```python
from build123d import *

# Parameters (mm, degrees)
BOSS_EXTRUDE1_DEPTH = 3
SKETCH2_W           = 78
SKETCH2_H           = 45
CUT_EXTRUDE1_DEPTH  = 10
FILLET1_R           = 10
CUT_EXTRUDE2_DEPTH  = 10


with BuildPart() as part:
    # Sketch1 → Boss-Extrude1 (new body)
    with BuildSketch(Plane(origin=(0, 0, 0), x_dir=(1, 0, 0), z_dir=(0, 1, 0))):
        Polygon((0, 0), (0, 75.000000004), (300, 65), (300, 0), align=None)
    boss_extrude1 = extrude(amount=BOSS_EXTRUDE1_DEPTH)

    # Mirror1: Boss-Extrude1 across Front Plane
    add(boss_extrude1.mirror(Plane.XY))

    # Sketch2 → Cut-Extrude1 (cut)
    with BuildSketch(Plane(origin=(0, 3, 0), x_dir=(1, 0, 0), z_dir=(0, 1, 0))):
        with Locations((55.5, 0)):
            Rectangle(SKETCH2_W, SKETCH2_H)
        with Locations((150, 0)):
            Rectangle(SKETCH2_W, SKETCH2_H)
        with Locations((244.5, 0)):
            Rectangle(SKETCH2_W, SKETCH2_H)
    extrude(amount=-CUT_EXTRUDE1_DEPTH, mode=Mode.SUBTRACT)

    # Fillet1
    fillet1_edges = [part.edges().sort_by_distance(p)[0] for p in [
        (16.5, 1.5, 22.5),
        (16.5, 1.5, -22.5),
        (94.5, 1.5, -22.5),
        (94.5, 1.5, 22.5),
        (111, 1.5, 22.5),
        (111, 1.5, -22.5),
        (189, 1.5, -22.5),
        (189, 1.5, 22.5),
        (205.5, 1.5, 22.5),
        (205.5, 1.5, -22.5),
        (283.5, 1.5, -22.5),
        (283.5, 1.5, 22.5),
    ]]
    fillet(fillet1_edges, radius=FILLET1_R)

    # Sketch3 → Cut-Extrude2 (cut)
    with BuildSketch(Plane(origin=(0, 3, 0), x_dir=(1, 0, 0), z_dir=(0, 1, 0))):
        with BuildLine():
            Line((12, 56.323336113), (12, 44))
            ThreePointArc((12, 44), (14.343145751, 38.343145751), (20, 36))
            Line((20, 36), (280, 36))
            ThreePointArc((280, 36), (285.656854249, 38.343145751), (288, 44))
            Line((288, 44), (288, 47.656669443))
            ThreePointArc((288, 47.656669443), (285.750310824, 53.218496969), (280.266518642, 55.652228699))
            Line((280.266518642, 55.652228699), (20.266518642, 64.318895369))
            ThreePointArc((20.266518642, 64.318895369), (14.438172474, 62.073646937), (12, 56.323336113))
        make_face()
    cut_extrude2 = extrude(amount=-CUT_EXTRUDE2_DEPTH, mode=Mode.SUBTRACT)

    # Mirror2: Cut-Extrude2 across plane
    add(cut_extrude2.mirror(Plane.XY), mode=Mode.SUBTRACT)


solid = part.part
```
Work out the finished part from the listing and answer in its coordinate system (mm). Coordinates: 2 decimals unless noted, no trailing zeros. Loops run counter-clockwise (first coordinate to the right, second up) from the corner with the lowest first, then second, coordinate; pieces in that order, holes last.
1) Section A-A (x = 209.5) is taken. Give the vertices of the cut face in (y, z).
Results:
outline: (0, -68.02) - (3, -68.02) - (3, -58.01) - (0, -58.01) - close; (0, -36) - (3, -36) - (3, -20.5) - (0, -20.5) - close; (0, 20.5) - (3, 20.5) - (3, 36) - (0, 36) - close; (0, 58.01) - (3, 58.01) - (3, 68.02) - (0, 68.02) - close
2) Section C-C (x = 167) is taken. Give the vertices of the cut face in (y, z), plus the area to 3 significant figures.
Results:
outline: (0, -69.43) - (3, -69.43) - (3, -59.43) - (0, -59.43) - close; (0, -36) - (3, -36) - (3, -22.5) - (0, -22.5) - close; (0, 22.5) - (3, 22.5) - (3, 36) - (0, 36) - close; (0, 59.43) - (3, 59.43) - (3, 69.43) - (0, 69.43) - close
area: 141 mm2
3) For a pull along Z with two mould halves and no side action, classify faces 1 (the flat face through (152, 3, -32)), 2 (the cylindrical face through (14.503, 1.521, 62.136)) as +Z half, -Z half, draft (parallel to the pull), parting line (faces both ways), or undercut.
Results:
face 1: draft
face 2: undercut
4) Flat-ended cylindrical pins translate along their axes: pin 1 (1.5 mm diameter, centred on x = 160, y = 2, fed in from +Z); pin 2 (1 mm diameter, centred on x = 137.5, y = 2, fed in from -Z); pin 3 (0.9 mm diameter, centred on x = 159.5, y = 2, fed in from -Z). Find the tip coordinate at first contact, or state that the pin passes through.
Results:
pin 1: stops at z = 69.69
pin 2: stops at z = -70.43
pin 3: stops at z = -69.7
5) Section B-B (y = 2.55) is taken. Give the number of separate pieces and of enclosed holes in the cut face, plus the area to 3 significant figures.
Results:
separate pieces: 1
enclosed holes: 5
area: 18,600 mm2
6) Consider probe 1 along X at (y, z) = (1, 7); probe 2 along Z at (x, y) = (154, 1.2); probe 3 along Z at (x, y) = (165, 1.35). Determine where each line is inside the solid, lowest interval first.
Results:
probe 1: x = 0 to 16.5, 94.5 to 111, 189 to 205.5, 283.5 to 300
probe 2: z = -69.87 to -59.86, -36 to -22.5, 22.5 to 36, 59.86 to 69.87
probe 3: z = -69.5 to -59.49, -36 to -22.5, 22.5 to 36, 59.49 to 69.5
